```python
from build123d import *

# Parameters (mm, degrees)
F2_R     = 12.7
F3_DEPTH = 76.2
F4_R     = 5.08


# Not quite as in the source:
# - a feature names something its author has since deleted; it is built from what else it names


with BuildPart() as f1:
    # F0 (on Front) → F1 (revolve)
    with BuildSketch(Plane.XZ):
        Polygon((0, -45.9611259629), (66.641533635, -45.9611259629), (25.5837057043, 10.3556019993), (25.5837057043, 75.9213268757), (0, 75.5790621042), align=None)
    revolve(axis=Axis((0, 0, 14.8089680707), (0, 0, -1)))

    # F2 (on Top) → F3 (cut, symmetric)
    with BuildSketch(Plane.XY):
        Circle(F2_R)
    extrude(amount=F3_DEPTH, both=True, mode=Mode.SUBTRACT)

    # F4
    f4_edges = [f1.edges().sort_by_distance(p)[0] for p in [
        (-66.641534, 0, -45.961126),
    ]]
    fillet(f4_edges, radius=F4_R)


solid = f1.part
```
Could you check a few things on this model? Use its own coordinates, in mm. Coordinates: 2 decimals unless noted, no trailing zeros. Write each loop counter-clockwise with the first axis right and the second up, starting at its lowest first coordinate (ties: lowest second). Pieces come first, ordered by that corner, then holes. Notation, with made-up numbers: (60, 57) -> (89, 57) arc R20 ccw to (89, 87) -> close; hole circle Ø7 at (44.5, 10.25). An arc over 180 degrees is marked (long way). Write item = value, one per line. Start each with the question number.
(1) I want a section at C-C (z = 27.5). Please give me the cut outline in (x, y).
(2) We'd pull the mould along Y, two halves only. Please class faces 1 (the face through (-5.916, 26.643, 8.013)), 2 (the face through (1, -13, -45.961)), 3 (the face through (-2.75, -12.4, 15.75)): released by +Y, released by -Y, zero draft, split by the parting line, or undercut.
(3) I want a section at A-A (y = 0). Please give me the cut outline in (x, z), plus the area to 3 significant figures.
(4) Will these pins go through, and if not, where does the flat tip stop? pin 1 (1 mm diameter, centred on x = 6.5, z = 19, fed in from +Y); pin 2 (6 mm diameter, centred on x = -29, z = 39, fed in from +Y); pin 3 (6 mm diameter, centred on x = 16, z = 57, fed in from -Y); pin 4 (3 mm diameter, centred on x = 48.5, y = 40, fed in from +Z).
(5) I need wall thicknesses on line 1 (Y direction, x = 0, z = 49); line 2 (X direction, y = 10, z = 60); line 3 (Y direction, x = -11, z = 39). Which ranges of each line are inside material? Lowest first, please. Write a range as [from, to].
Result set:
q1.outline = circle Ø51.17 at (0, 0); hole circle Ø25.4 at (0, 0)
q2.face_1 = split by the parting line
q2.face_2 = zero draft
q2.face_3 = undercut
q3.outline = (-60.76, -37.89) arc R5.08 ccw to (-56.65, -45.96) -> (-12.7, -45.96) -> (-12.7, 75.75) -> (-25.58, 75.92) -> (-25.58, 10.36) -> close; (12.7, -45.96) -> (56.65, -45.96) arc R5.08 ccw to (60.76, -37.89) -> (25.58, 10.36) -> (25.58, 75.92) -> (12.7, 75.75) -> close
q3.area = 5,410 mm2
q4.pin_1 = 24.87
q4.pin_2 = through
q4.pin_3 = -22.03
q4.pin_4 = -38.99
q5.line_1 = [-25.58, -12.7], [12.7, 25.58]
q5.line_2 = [-23.55, -7.83], [7.83, 23.55]
q5.line_3 = [-23.1, -6.35], [6.35, 23.1]
